from build123d import *

# Parameters (mm, degrees)
SKETCH1_W           = 1250
SKETCH1_H           = 1093
BOSS_EXTRUDE1_DEPTH = 1
CUT_EXTRUDE1_DEPTH  = 10
FILLET2_R           = 3
SKETCH3_R           = 1.75
CUT_EXTRUDE2_DEPTH  = 10


with BuildPart() as part:
    # Sketch1 → Boss-Extrude1 (new body)
    with BuildSketch(Plane(origin=(0, 0, 0), x_dir=(1, 0, 0), z_dir=(0, 1, 0))):
        Rectangle(SKETCH1_W, SKETCH1_H)
    extrude(amount=BOSS_EXTRUDE1_DEPTH)

    # Sketch2 → Cut-Extrude1 (cut)
    with BuildSketch(Plane(origin=(0, 1, 0), x_dir=(1, 0, 0), z_dir=(0, 1, 0))):
        Polygon((-334, 256), (-260, 256), (-260, 384), (-340, 384), (-340, 296), (-334, 296), align=None)
    extrude(amount=-CUT_EXTRUDE1_DEPTH, mode=Mode.SUBTRACT)

    # Fillet2
    fillet2_edges = [part.edges().sort_by_distance(p)[0] for p in [
        (-260, 0.5, -256),
        (-334, 0.5, -256),
        (-334, 0.5, -296),
        (-340, 0.5, -296),
        (-340, 0.5, -384),
        (-260, 0.5, -384),
    ]]
    fillet(fillet2_edges, radius=FILLET2_R - 0.0001)  # a hair under: the kernel refuses the full size

    # Sketch3 → Cut-Extrude2 (cut)
    with BuildSketch(Plane(origin=(0, 1, 0), x_dir=(1, 0, 0), z_dir=(0, 1, 0))):
        with Locations(Location((-264, 389, 0), (0, 0, 270))):
            Circle(SKETCH3_R)
        with Locations(Location((-328, 389, 0), (0, 0, 270))):
            Circle(SKETCH3_R)
        with Locations(Location((-338, 275, 0), (0, 0, 270))):
            Circle(SKETCH3_R)
        with Locations(Location((-264, 251, 0), (0, 0, 270))):
            Circle(SKETCH3_R)
    extrude(amount=-CUT_EXTRUDE2_DEPTH, mode=Mode.SUBTRACT)


solid = part.part
Work out the finished part from the listing and answer in its coordinate system (mm). Give positions to 0.01 mm unless a question says otherwise; leave off trailing zeros. Order: outer loops, then holes, each group sorted by start corner. A loop starts at its lowest first (then second) coordinate and runs counter-clockwise, first axis right, second up. Notation, with made-up numbers: (35.5, -31.5) - (55.5, -31.5) arc R21 cw to (55.5, -16.5) - close; hole circle Ø11 at (-24.75, -10.5). An arc over 180 degrees is marked (long way). Answer as CSV lines item,"result". Start each with the question number.
Q1. Given pin 1 Ø8 at (x, z) = (488.5, 434) entering from -Y; pin 2 Ø3 at (x, z) = (-338, -275) entering from +Y, each flat-ended and moving along its own axis, determine where each tip first touches the part or whether it passes through.
Q2. Find the intervals of material crossed by L1, parallel to Z at x = -338, y = 0.85; L2, parallel to Z at x = -264, y = 0.45; L3, parallel to Z at x = -328, y = 0.75, in increasing order. Write a range as [from, to].
Q3. The part is cut by section A-A (z = -321). Write down the section's boundary in (x, y), then the cut area to 3 significant figures.
Check result:
1,pin 1,"stops at y = 0"
1,pin 2,"passes through"
2,L1,"z = [-546.5, -383.83], [-296.17, -276.75], [-273.25, 546.5]"
2,L2,"z = [-546.5, -390.75], [-387.25, -384], [-256, -252.75], [-249.25, 546.5]"
2,L3,"z = [-546.5, -390.75], [-387.25, -384], [-256, 546.5]"
3,outline,"(-625, 0) - (-340, 0) - (-340, 1) - (-625, 1) - close; (-260, 0) - (625, 0) - (625, 1) - (-260, 1) - close"
3,area,"1,170 mm²"
